```python
from build123d import *

# Parameters (mm, degrees)
F1_DEPTH = 63.5
F2_DEPTH = 31.75
F0_W     = 25.4
F0_H     = 8.5634328214
F3_DEPTH = 25.4
F5_R     = 5.08


with BuildPart() as f1:
    # F0 (on Front) → F1 (new body, symmetric)
    with BuildSketch(Plane.XZ):
        Polygon((50.8, -15.875), (50.8, 15.875), (31.75, 15.875), (-50.8, 15.875), (-50.8, -15.875), align=None)
    extrude(amount=F1_DEPTH, both=True)

    # F0 (on Front) → F2 (join, symmetric)
    with BuildSketch(Plane.XZ):
        with BuildLine():
            Line((-50.8, 15.875), (31.75, 15.875))
            Line((31.75, 15.875), (31.75, 63.5))
            ThreePointArc((31.75, 63.5), (41.7112794582, 87.9247473214), (65.9128221454, 98.4166824014))
            add(Edge.make_bspline(
                [(-50.8, 15.875), (-20.8947578711, 55.0768055935), (18.9205500182, 97.6768686264), (65.9128221454, 98.4166824014)],
                knots=[0, 0, 0, 0, 142.8073833678, 142.8073833678, 142.8073833678, 142.8073833678], degree=3))
        make_face()
        with BuildLine():
            Line((31.75, 15.875), (50.8, 15.875))
            Line((50.8, 15.875), (50.8, 63.5))
            ThreePointArc((50.8, 63.5), (55.4496798487, 74.7253201513), (66.675, 79.375))
            Line((66.675, 79.375), (69.6957821591, 79.375))
            Line((69.6957821591, 79.375), (69.6957821591, 98.425))
            Line((69.6957821591, 98.425), (66.675, 98.425))
            add(Edge.make_bspline(
                [(65.9128221454, 98.4166824014), (66.1666721422, 98.4206788398), (66.4207315707, 98.4234537508), (66.675, 98.425)],
                knots=[142.8073833678, 142.8073833678, 142.8073833678, 142.8073833678, 143.5788219934, 143.5788219934, 143.5788219934, 143.5788219934], degree=3))
            ThreePointArc((65.9128221454, 98.4166824014), (41.7112794582, 87.9247473214), (31.75, 63.5))
            Line((31.75, 63.5), (31.75, 15.875))
        make_face()
    extrude(amount=F2_DEPTH, both=True)

    # F0 (on Front) → F3 (join, symmetric)
    with BuildSketch(Plane.XZ):
        with Locations((82.3957821591, 75.0932835893)):
            Rectangle(F0_W, F0_H)
        Polygon((69.6957821591, 98.425), (69.6957821591, 79.375), (95.0957821591, 79.375), (95.0957821591, 104.775), (69.6957821591, 104.775), align=None)
    extrude(amount=F3_DEPTH, both=True)

    # F0 (on Front) → F4 (revolve)
    with BuildSketch(Plane.XZ):
        Polygon((95.0957821591, 104.775), (95.0957821591, 79.375), (95.0957821591, 70.8115671786), (120.4957821591, 70.8115671786), (120.4957821591, 104.775), align=None)
    revolve(axis=Axis((95.0957821591, 0, 87.7932835893), (0, 0, 1)))

    # F5
    f5_edges = [f1.edges().sort_by_distance(p)[0] for p in [
        (50.8, -63.5, 0),
        (-50.8, -63.5, 0),
        (-50.8, 63.5, 0),
        (50.8, 63.5, 0),
    ]]
    fillet(f5_edges, radius=F5_R)


solid = f1.part
```
Build history of the part. All positions in model axes, mm. A direction names the side the tool comes from. Coordinates: 2 decimals unless noted, no trailing zeros. Write each loop counter-clockwise with the first axis right and the second up, starting at its lowest first coordinate (ties: lowest second). Pieces come first, ordered by that corner, then holes.
1. Drop flat-ended pins along their axis: pin 1 (9.5 mm diameter, centred on x = -16.5, y = -52.5, fed in from +Z) (3 decimals); pin 2 (25 mm diameter, centred on x = 33.5, z = 42, fed in from +Y); pin 3 (1.9 mm diameter, centred on y = -8, z = 100.5, fed in from -X). Give the stop position or say it passes through.
Answer block:
pin 1: stops at z = 15.875
pin 2: stops at y = 31.75
pin 3: stops at x = 69.7
2. 3-axis set-ups, long thin cutter, end or side, ignore diameter. For faces 1 (the flat face through (69.696, 29, 89)), 2 (the flat face through (1, -48, 15.875)), 3 (the flat face through (82, -25.4, 88)): which of +Z, -Z, +X, -X, +Y, -Y reach the whole face in a straight line?
Answer block:
face 1: +Z, -Z, +X, +Y
face 2: +Z, +X, -X, -Y
face 3: +Z, -Z, +X, -Y
3. Band-saw the part on B-B, the plane y = 36. Give the cut face in (x, z) (3 decimals), and give its area (3 significant figures).
Answer block:
outline: (-50.8, -15.875) - (50.8, -15.875) - (50.8, 15.875) - (-50.8, 15.875) - close
area: 3,230 mm2
4. Band-saw the part on A-A, the plane z = 8. Give the cut face in (x, y).
Answer block:
outline: (-50.8, -58.42) arc R5.08 ccw to (-45.72, -63.5) - (45.72, -63.5) arc R5.08 ccw to (50.8, -58.42) - (50.8, 58.42) arc R5.08 ccw to (45.72, 63.5) - (-45.72, 63.5) arc R5.08 ccw to (-50.8, 58.42) - close
5. Pull direction X, two halves, no side cores. Call faces 4 (the flat face through (-50.8, -1, 0)), 5 (the flat face through (69.696, 0, 75)), 6 (the flat face through (-1, -63.5, 0)): released by +X, released by -X, zero draft, split by the parting line, or undercut.
Answer block:
face 4: released by -X
face 5: undercut
face 6: zero draft
6. Drill centre lines: probe 1 along Z at (x, y) = (34, 51) (3 decimals); probe 2 along Y at (x, z) = (-13.5, 57.5); probe 3 along X at (y, z) = (-41, 8.5). Where is each one in solid material? Low to high.
Answer block:
probe 1: z = -15.875 to 15.875
probe 2: y = -31.75 to 31.75
probe 3: x = -50.8 to 50.8
7. Band-saw the part on C-C, the plane x = 109. Give the cut face in (y, z) (3 decimals), and give its area (3 significant figures).
Answer block:
outline: (-21.256, 70.812) - (21.256, 70.812) - (21.256, 104.775) - (-21.256, 104.775) - close
area: 1,440 mm2
